Verification items for this drawing (mm, ordinates from the low corner). Give positions to 0.01 mm unless a question says otherwise; leave off trailing zeros. Order: outer loops, then holes, each group sorted by start corner. A loop starts at its lowest first (then second) coordinate and runs counter-clockwise, first axis right, second up. Notation, with made-up numbers: M -36,38 L -9,38 A25 cw -9,71 Z; hole C -29,-23.75 d4. An arc over 180 degrees is marked long. Answer as a JSON object with one key per item and string values.
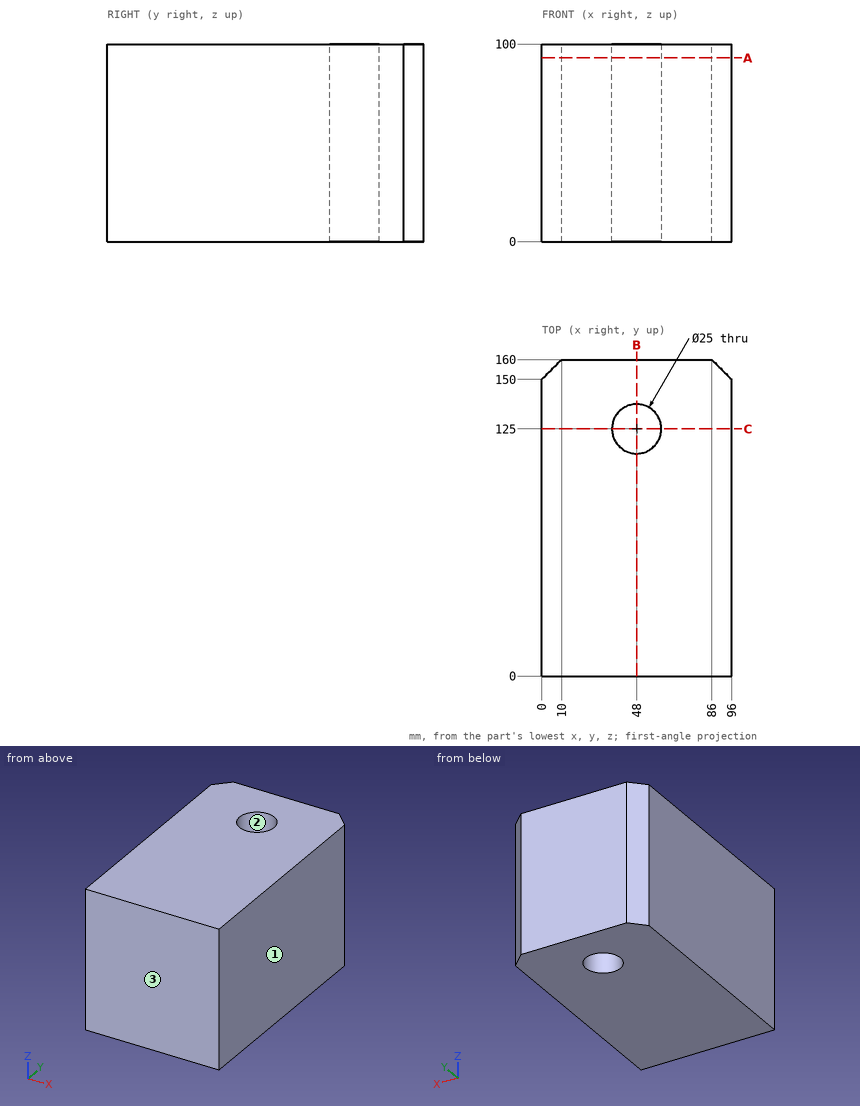
Q1. Gauge pin test, flat end, axial feed: pin 1 Ø4 at (y, z) = (98, 38) entering from -X. Record the tip position at first contact, or that the pin passes through.
Resolved:
{"pin 1": "stops at x = 0"}
Q2. Section check B-B on x = 48. Record the cut outline in (y, z).
Resolved:
{"outline": "M 0,0 L 112.5,0 L 112.5,100 L 0,100 Z; M 137.5,0 L 160,0 L 160,100 L 137.5,100 Z"}
Q3. Section check A-A on z = 93. Record the cut outline in (x, y).
Resolved:
{"outline": "M 0,0 L 96,0 L 96,150 L 86,160 L 10,160 L 0,150 Z; hole C 48,125 d25"}
Q4. Section check C-C on y = 125. Record the cut outline in (x, z).
Resolved:
{"outline": "M 0,0 L 35.5,0 L 35.5,100 L 0,100 Z; M 60.5,0 L 96,0 L 96,100 L 60.5,100 Z"}
Q5. Release check for a two-part mould opening along Y. For the marked faces 1, 2 and 3 record: +Y half, -Y half, draft (parallel to the pull), parting line (faces both ways), or undercut.
Resolved:
{"face 1": "draft", "face 2": "undercut", "face 3": "-Y half"}
Q6. Material ranges on L1, parallel to Y at x = 48, z = 40; L2, parallel to X at y = 128, z = 76; L3, parallel to Y at x = 55, z = 77.5, recorded low to high.
Resolved:
{"L1": "y = 0 to 112.5, 137.5 to 160", "L2": "x = 0 to 35.87, 60.13 to 96", "L3": "y = 0 to 114.64, 135.36 to 160"}
